Autodesk Inventor part; units mm, degrees
ref_plane "YZ Plane" through (0, 0, 0) normal (1, 0, 0) x (0, 1, 0)
ref_plane "XZ Plane" through (0, 0, 0) normal (0, 1, 0) x (-1, 0, 0)
ref_plane "XY Plane" through (0, 0, 0) normal (0, 0, 1) x (1, 0, 0)
sketch "Sketch1" plane through (0, 0, 0) normal (0, 0, 1) x (1, 0, 0)
  line L0 (0, 0) -> (-25.4, 0)
  line L1 (-25.4, 0) -> (-25.4, -25.4)
  line L2 (-25.4, -25.4) -> (0, -25.4)
  line L3 (0, -25.4) -> (0, 0)
  line L4 (-3.175, -22.225) -> (-22.225, -22.225)
  line L5 (-22.225, -22.225) -> (-22.225, -3.175)
  line L6 (-22.225, -3.175) -> (-3.175, -3.175)
  line L7 (-3.175, -3.175) -> (-3.175, -22.225)
  dimension "d0" = 25.4
  dimension "d1" = 25.4
  dimension "d2" = 3.175
extrude "Extrusion1" add sketch "Sketch1" along normal blind 228.6
sketch "Sketch2" plane through (-25.4, -25.4, 0) normal (0, -1, 0) x (1, 0, 0)
  circle A0 centre (12.7, 190.5) radius 3.175
  line L0 (0, 228.6) -> (25.4, 228.6)
  line L1 (0, 0) -> (0, 228.6)
  circle A1 centre (12.7, 12.7) radius 3.175
  circle A2 centre (12.7, 57.15) radius 3.175
  line L2 (0, 0) -> (25.4, 0)
  dimension "d5" = 6.35
  dimension "d6" = 38.1
  dimension "d7" = 12.7
  dimension "d10" = 6.35
  dimension "d11" = 12.7
  dimension "d12" = 44.45
  dimension "d13" = 12.7
  dimension "d14" = 12.7
extrude "Extrusion2" cut sketch "Sketch2" against normal blind 152.4
properties part number "15102898-16-A-0205" material "Aluminum 6061"
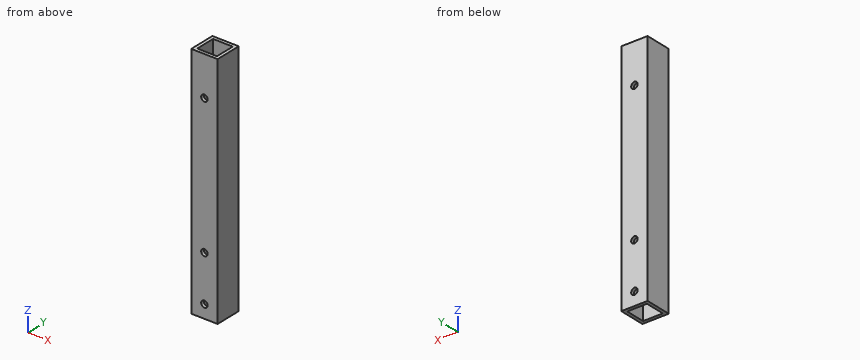
Source: CAD feature listing. Evaluate the final solid. Frame: model axes, mm. Coordinates: 2 decimals unless noted, no trailing zeros. Loops run counter-clockwise (first coordinate to the right, second up) from the corner with the lowest first, then second, coordinate; pieces in that order, holes last. Notation, with made-up numbers: (-30.75, 38) - (23.25, 38) arc R32 cw to (23.25, 74) - close; hole circle Ø7 at (65, 37). An arc over 180 degrees is marked (long way). Answer as CSV lines item,"result".
1. Contact query for a flat-ended pin moving along its axis: pin 1 (5.5 mm diameter, centred on x = -12.7, z = 12.7, fed in from +Y). Output: stop coordinate, or through.
Established:
pin 1,"passes through"
2. Section A-A (y = -16.75). Return loops of the section in (x, z) (3 decimals), then the cut area to 3 significant figures.
Established:
outline,"(-25.4, 0) - (-22.225, 0) - (-22.225, 228.6) - (-25.4, 228.6) - close; (-3.175, 0) - (0, 0) - (0, 228.6) - (-3.175, 228.6) - close"
area,"1,450 mm2"
3. Section B-B (z = 57.15). Return loops of the section in (x, y) (3 decimals), then the cut area to 3 significant figures.
Established:
outline,"(-25.4, -25.4) - (-15.875, -25.4) - (-15.875, -22.225) - (-22.225, -22.225) - (-22.225, -3.175) - (-15.875, -3.175) - (-15.875, 0) - (-25.4, 0) - close; (-9.525, -25.4) - (0, -25.4) - (0, 0) - (-9.525, 0) - (-9.525, -3.175) - (-3.175, -3.175) - (-3.175, -22.225) - (-9.525, -22.225) - close"
area,"242 mm2"
4. Ray query, line 1 (Z direction, x = -12.7, y = -1.2) (3 decimals); line 2 (Y direction, x = -21.25, z = 123) (3 decimals). Return the intervals inside material, ascending.
Established:
line 1,"z = 0 to 9.525, 15.875 to 53.975, 60.325 to 187.325, 193.675 to 228.6"
line 2,"y = -25.4 to -22.225, -3.175 to 0"
5. Section C-C (x = -12.7). Count the separate pieces of the cut face and the enclosed holes in it, then the cut area to 3 significant figures.
Established:
separate pieces,"8"
enclosed holes,"0"
area,"1,330 mm2"
